Model file for the job. Use its own axes, mm. A direction names the side the tool comes from. Coordinates: 2 decimals unless noted, no trailing zeros. Write each loop counter-clockwise with the first axis right and the second up, starting at its lowest first coordinate (ties: lowest second). Pieces come first, ordered by that corner, then holes. Notation, with made-up numbers: (77, 51.5) -> (125, 51.5) arc R10 cw to (125, 55.5) -> close; hole circle Ø4 at (-16, 2.25). An arc over 180 degrees is marked (long way). Write item = value, one per line. Start each with the question number.
from build123d import *

# Parameters (mm, degrees)
F2_R      = 1.6002
F4_DEPTH  = 25.4
F5_DEPTH  = 25.4
F6_R      = 3.175
F7_DEPTH  = 5.08
F8_DEPTH  = 3.175
F9_R      = 1.5875
F10_DEPTH = 3.175
F12_D     = 1.5875
F12_DEPTH = 6.35
F12_TIP   = 0.4769331164


with BuildPart() as f1:
    # F0 (on Top) → F1 (revolve)
    with BuildSketch(Plane.XY):
        with BuildLine():
            Line((-3.556, -6.35), (-3.556, 0))
            Line((-3.556, 0), (-25.4, 0))
            ThreePointArc((-25.4, 0), (-28.575, -3.175), (-25.4, -6.35))
            Line((-25.4, -6.35), (-20.6502, -6.35))
            ThreePointArc((-20.6502, -6.35), (-21.7817122713, -3.6182877287), (-19.05, -4.7498))
            Line((-19.05, -4.7498), (-5.1562, -4.7498))
            ThreePointArc((-5.1562, -4.7498), (-4.6875122713, -5.8813122713), (-3.556, -6.35))
        make_face()
        with BuildLine():
            ThreePointArc((-19.05, -4.7498), (-21.7817122713, -3.6182877287), (-20.6502, -6.35))
            ThreePointArc((-20.6502, -6.35), (-19.5186877287, -5.8813122713), (-19.05, -4.7498))
        make_face()
    revolve(axis=Axis((0, -3.1282322016, 0), (0, -1, 0)))

    # F2
    f2_edges = [f1.edges().sort_by_distance(p)[0] for p in [
        (5.1562, -4.7498, 0),
    ]]
    fillet(f2_edges, radius=F2_R)

    # F3 (on face) → F4 (cut)
    with BuildSketch(Plane.XZ.offset(4.7498)):
        with BuildLine():
            ThreePointArc((-2.4323813859, 9.0777709155), (0, 9.398), (2.4323813859, 9.0777709155))
            Line((2.4323813859, 9.0777709155), (4.1416223597, 15.4567450723))
            ThreePointArc((4.1416223597, 15.4567450723), (0, 16.002), (-4.1416223597, 15.4567450723))
            Line((-4.1416223597, 15.4567450723), (-2.4323813859, 9.0777709155))
        make_face()
    extrude(amount=-F4_DEPTH, mode=Mode.SUBTRACT)

    # F3 (on face) → F5 (cut)
    with BuildSketch(Plane.XZ.offset(4.7498)):
        with BuildLine():
            ThreePointArc((-9.0777709155, 2.4323813859), (-8.1389067448, 4.699), (-6.6453895296, 6.6453895296))
            Line((-6.6453895296, 6.6453895296), (-11.3151227125, 11.3151227125))
            ThreePointArc((-11.3151227125, 11.3151227125), (-13.8581385114, 8.001), (-15.4567450723, 4.1416223597))
            Line((-15.4567450723, 4.1416223597), (-9.0777709155, 2.4323813859))
        make_face()
        with BuildLine():
            ThreePointArc((6.6453895296, 6.6453895296), (8.1389067448, 4.699), (9.0777709155, 2.4323813859))
            Line((9.0777709155, 2.4323813859), (15.4567450723, 4.1416223597))
            ThreePointArc((15.4567450723, 4.1416223597), (13.8581385114, 8.001), (11.3151227125, 11.3151227125))
            Line((11.3151227125, 11.3151227125), (6.6453895296, 6.6453895296))
        make_face()
        with BuildLine():
            ThreePointArc((9.0777709155, -2.4323813859), (8.1389067448, -4.699), (6.6453895296, -6.6453895296))
            Line((6.6453895296, -6.6453895296), (11.3151227125, -11.3151227125))
            ThreePointArc((11.3151227125, -11.3151227125), (13.8581385114, -8.001), (15.4567450723, -4.1416223597))
            Line((15.4567450723, -4.1416223597), (9.0777709155, -2.4323813859))
        make_face()
        with BuildLine():
            ThreePointArc((2.4323813859, -9.0777709155), (0, -9.398), (-2.4323813859, -9.0777709155))
            Line((-2.4323813859, -9.0777709155), (-4.1416223597, -15.4567450723))
            ThreePointArc((-4.1416223597, -15.4567450723), (0, -16.002), (4.1416223597, -15.4567450723))
            Line((4.1416223597, -15.4567450723), (2.4323813859, -9.0777709155))
        make_face()
        with BuildLine():
            ThreePointArc((-6.6453895296, -6.6453895296), (-8.1389067448, -4.699), (-9.0777709155, -2.4323813859))
            Line((-9.0777709155, -2.4323813859), (-15.4567450723, -4.1416223597))
            ThreePointArc((-15.4567450723, -4.1416223597), (-13.8581385114, -8.001), (-11.3151227125, -11.3151227125))
            Line((-11.3151227125, -11.3151227125), (-6.6453895296, -6.6453895296))
        make_face()
    extrude(amount=-F5_DEPTH, mode=Mode.SUBTRACT)

    # F6 (on face) → F7 (join)
    with BuildSketch(Plane.XZ.offset(6.35)):
        with Locations((17.78, 0)):
            Circle(F6_R)
    extrude(amount=-F7_DEPTH)

    # F6 (on face) → F8 (join)
    with BuildSketch(Plane.XZ.offset(6.35)):
        with BuildLine():
            ThreePointArc((20.6502, 0), (20.6372419344, 0.7314406207), (20.598384, 1.4619632788))
            ThreePointArc((20.598384, 1.4619632788), (14.605, 0), (20.598384, -1.4619632788))
            ThreePointArc((20.598384, -1.4619632788), (20.6372419344, -0.7314406207), (20.6502, 0))
        make_face()
        with BuildLine():
            ThreePointArc((20.598384, -1.4619632788), (20.8645578451, -0.7524147128), (20.955, 0))
            ThreePointArc((20.955, 0), (20.8645578451, 0.7524147128), (20.598384, 1.4619632788))
            ThreePointArc((20.598384, 1.4619632788), (20.6372419344, 0.7314406207), (20.6502, 0))
            ThreePointArc((20.6502, 0), (20.6372419344, -0.7314406207), (20.598384, -1.4619632788))
        make_face()
    extrude(amount=F8_DEPTH)

    # F9 (on face) → F10 (join)
    with BuildSketch(Plane.XZ.offset(9.525)):
        with Locations((17.78, 0)):
            Circle(F9_R)
    extrude(amount=F10_DEPTH)

    # F12
    with Locations(Plane.XZ.offset(12.7)):
        with Locations((17.78, 0)):
            Hole(F12_D / 2, depth=F12_DEPTH)
            with Locations((0, 0, -(F12_DEPTH + F12_TIP / 2))):  # 118° drill point
                Cone(0, F12_D / 2, F12_TIP, mode=Mode.SUBTRACT)


solid = f1.part
(1) 3-axis set-ups, long thin cutter, end or side, ignore diameter. For faces 4 (the face through (16, -9.525, -1)), 5 (the face through (0, -2, -16)): which of +Z, -Z, +X, -X, +Y, -Y reach the whole face in a straight line?
(2) Saw through at A-A (y = -1). Give the cut face in (x, z).
(3) Mould opens along Z. For faces 1 (the face through (18, -12.7, 1)), 2 (the face through (-9, -2, -9)), 3 (the face through (-13.887, -2.408, -7.95)) say: released by +Z, released by -Z, zero draft, split by the parting line, or undercut.
(4) Saw through at B-B (x = 0). State how many separate pieces and enclosed holes the cut face has, then the cut area to 3 significant figures.
(5) Saw through at C-C (y = -10.5). Give the cut face in (x, z) (1 decimal).
(6) Drop flat-ended pins along their axis: pin 1 Ø1.5 at (x, y) = (2, -1.5) entering from -Z; pin 2 Ø15 at (x, z) = (5, 7.5) entering from -Y; pin 3 Ø6 at (y, z) = (-8.5, 6) entering from -X. Give the stop position or say it passes through.
(7) Drill centre lines: line 1 along Z through (x, y) = (-13.5, -2.75); line 2 along X through (y, z) = (-4.5, -4.5); line 3 along Y through (x, z) = (5.5, -14). Where is each one in solid material? Low to high.
Returned:
q1.face_4 = -Y
q1.face_5 = +Y, -Y
q2.outline = circle Ø55.43 at (0, 0); hole (-15.46, -4.14) arc R16 ccw to (-11.32, -11.32) -> (-6.65, -6.65) arc R9.4 cw to (-9.08, -2.43) -> close; hole (-15.46, 4.14) -> (-9.08, 2.43) arc R9.4 cw to (-6.65, 6.65) -> (-11.32, 11.32) arc R16 ccw to start; hole (-4.14, -15.46) arc R16 ccw to (4.14, -15.46) -> (2.43, -9.08) arc R9.4 cw to (-2.43, -9.08) -> close; hole (-4.14, 15.46) -> (-2.43, 9.08) arc R9.4 cw to (2.43, 9.08) -> (4.14, 15.46) arc R16 ccw to start; hole circle Ø7.11 at (0, 0); hole (6.65, -6.65) -> (11.32, -11.32) arc R16 ccw to (15.46, -4.14) -> (9.08, -2.43) arc R9.4 cw to start; hole (6.65, 6.65) arc R9.4 cw to (9.08, 2.43) -> (15.46, 4.14) arc R16 ccw to (11.32, 11.32) -> close
q3.face_1 = zero draft
q3.face_2 = undercut
q3.face_3 = undercut
q4.separate_pieces = 4
q4.enclosed_holes = 0
q4.area = 200 mm2
q5.outline = circle Ø3.2 at (17.8, 0); hole circle Ø1.6 at (17.8, 0)
q6.pin_1 = -28.37
q6.pin_2 = -6.35
q6.pin_3 = -26.96
q7.line_1 = -25.15 to -8.59, -3.62 to 3.62, 8.59 to 25.15
q7.line_2 = -27.93 to -15.36, -8.25 to 8.25, 15.36 to 27.93
q7.line_3 = -4.75 to 0
